Read the model definition and answer for the solid it produces. Units are mm, in the model's axes. Coordinates: 2 decimals unless noted, no trailing zeros. Answer in a Markdown table with one row per item.
```python
from build123d import *

# Parameters (mm, degrees)
F0_R     = 2.0955
F1_DEPTH = 3.175


with BuildPart() as f1:
    # F0 (on Top) → F1 (new body)
    with BuildSketch(Plane.XY):
        with BuildLine():
            Line((3.81, 0), (0, 0))
            Line((0, 0), (0, -5.08))
            Line((0, -5.08), (1.7145, -5.08))
            ThreePointArc((1.7145, -5.08), (2.32825774, -3.59825774), (3.81, -2.9845))
            Line((3.81, -2.9845), (3.81, 0))
        make_face()
        with BuildLine():
            Line((101.6, 0), (3.81, 0))
            Line((3.81, 0), (3.81, -2.9845))
            ThreePointArc((3.81, -2.9845), (5.29174226, -3.59825774), (5.9055, -5.08))
            Line((5.9055, -5.08), (90.1827, -5.08))
            ThreePointArc((90.1827, -5.08), (92.2782, -2.9845), (94.3737, -5.08))
            Line((94.3737, -5.08), (101.6, -5.08))
            Line((101.6, -5.08), (101.6, 0))
        make_face()
        with BuildLine():
            Line((1.7145, -5.08), (0, -5.08))
            Line((0, -5.08), (0, -104.14))
            Line((0, -104.14), (3.81, -104.14))
            Line((3.81, -104.14), (3.81, -50.0634))
            Line((3.81, -50.0634), (3.81, -45.0469))
            ThreePointArc((3.81, -45.0469), (1.7145, -42.9514), (3.81, -40.8559))
            Line((3.81, -40.8559), (3.81, -7.1755))
            ThreePointArc((3.81, -7.1755), (2.32825774, -6.56174226), (1.7145, -5.08))
        make_face()
        with BuildLine():
            Line((101.6, -104.14), (101.6, -5.08))
            Line((101.6, -5.08), (94.3737, -5.08))
            ThreePointArc((94.3737, -5.08), (92.2782, -7.1755), (90.1827, -5.08))
            Line((90.1827, -5.08), (5.9055, -5.08))
            ThreePointArc((5.9055, -5.08), (5.29174226, -6.56174226), (3.81, -7.1755))
            Line((3.81, -7.1755), (3.81, -40.8559))
            ThreePointArc((3.81, -40.8559), (5.29174226, -41.46965774), (5.9055, -42.9514))
            ThreePointArc((5.9055, -42.9514), (5.29174226, -44.43314226), (3.81, -45.0469))
            Line((3.81, -45.0469), (3.81, -50.0634))
            Line((3.81, -50.0634), (3.81, -104.14))
            Line((3.81, -104.14), (101.6, -104.14))
        make_face()
        with Locations((17.7038, -98.2599)):
            Circle(F0_R, mode=Mode.SUBTRACT)
        with Locations((69.215, -93.2561)):
            Circle(F0_R, mode=Mode.SUBTRACT)
        with Locations((89.154, -82.2198)):
            Circle(F0_R, mode=Mode.SUBTRACT)
        with Locations((69.215, -65.4431)):
            Circle(F0_R, mode=Mode.SUBTRACT)
        with BuildLine():
            ThreePointArc((19.7993, -50.0634), (17.7038, -52.1589), (15.6083, -50.0634))
            ThreePointArc((15.6083, -50.0634), (17.7038, -47.9679), (19.7993, -50.0634))
        make_face(mode=Mode.SUBTRACT)
        with BuildLine():
            ThreePointArc((79.3877, -50.0634), (77.2922, -52.1589), (75.1967, -50.0634))
            ThreePointArc((75.1967, -50.0634), (77.2922, -47.9679), (79.3877, -50.0634))
        make_face(mode=Mode.SUBTRACT)
        with BuildLine():
            ThreePointArc((94.3737, -42.9514), (92.2782, -45.0469), (90.1827, -42.9514))
            ThreePointArc((90.1827, -42.9514), (92.2782, -40.8559), (94.3737, -42.9514))
        make_face(mode=Mode.SUBTRACT)
    extrude(amount=-F1_DEPTH)


solid = f1.part
```
1. The mould has two halves that part along X. Classify faces 1 (the flat face through (101.6, -53, -2)), 2 (the flat face through (50, -51, -3.175)), 3 (the flat face through (0, -51, -2)), 4 (the cylindrical face through (94.37, -42.86, -1.57)): pulls with the +X half, pulls with the -X half, needs draft (parallel to the pull), parting line crosses it, or undercut.
A:
| item | result |
|---|---|
| face 1 | pulls with the +X half |
| face 2 | needs draft |
| face 3 | pulls with the -X half |
| face 4 | undercut |
2. Given pin 1 Ø2.5 at (x, y) = (69.22, -93.26) entering from +Z, flat-ended and moving along its own axis, determine where the tip first touches the part or whether it passes through.
A:
| item | result |
|---|---|
| pin 1 | passes through |
3. Find the intervals of material crossed by probe 1 along X at (y, z) = (-43, -2.75); probe 2 along Y at (x, z) = (18, -0.7); probe 3 along Y at (x, z) = (19, -1), in increasing order.
A:
| item | result |
|---|---|
| probe 1 | x = 0 to 1.72, 5.9 to 90.18, 94.37 to 101.6 |
| probe 2 | y = -104.14 to -100.33, -96.19 to -52.14, -47.99 to 0 |
| probe 3 | y = -104.14 to -99.91, -96.61 to -51.71, -48.42 to 0 |
